```python
from build123d import *

# Parameters (mm, degrees)
F0_W     = 75.5904
F0_H     = 25.2222
F0_W_2   = 22.2504
F0_H_2   = 12.5222
F1_DEPTH = 0.9652
F2_W     = 31.75
F2_H     = 17.78
F3_DEPTH = 0.3048


with BuildPart() as f1:
    # F0 (on Top) → F1 (new body)
    with BuildSketch(Plane.XY):
        Rectangle(F0_W, F0_H)
        Rectangle(F0_W_2, F0_H_2, mode=Mode.SUBTRACT)
    extrude(amount=F1_DEPTH)

    # F2 (on face) → F3 (cut)
    with BuildSketch(Plane.XY.offset(0.9652)):
        Rectangle(F2_W, F2_H)
    extrude(amount=-F3_DEPTH, mode=Mode.SUBTRACT)


solid = f1.part
```
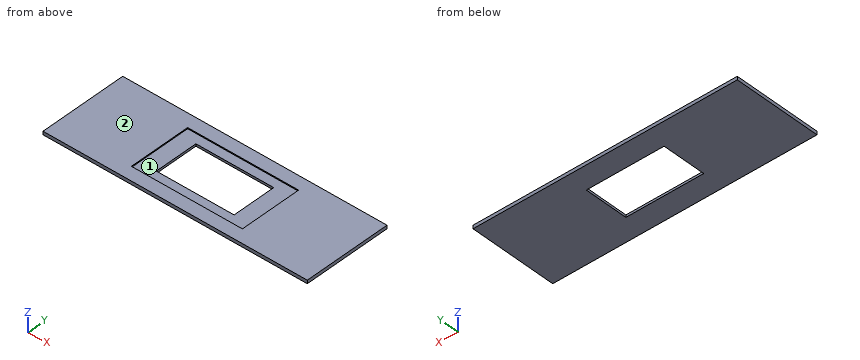
Verification items for the finished model (mm, model axes). Face numbers are marked on the shaded views. Round coordinates to 2 decimals unless told otherwise and drop trailing zeros. Order: outer loops, then holes, each group sorted by start corner. A loop starts at its lowest first (then second) coordinate and runs counter-clockwise, first axis right, second up. Notation, with made-up numbers: (-37.5, 76) -> (14.5, 76) arc R16 ccw to (14.5, 106) -> close; hole circle Ø5 at (12, -35). An arc over 180 degrees is marked (long way). Put each result on its own line as item: value. Start each with the question number.
(1) Depth check by flat-ended pin: pin 1 Ø1 at (x, y) = (-21, 0.5) entering from -Z. Enter the tip coordinate at first touch or a pass-through.
(2) Section check A-A (y = 2.75). Enter the section's corners in (x, z) (3 decimals), then the cut area to 3 significant figures.
(3) Draft check along Y on the marked faces 1 and 2. Enter one of: +Y half, -Y half, draft (parallel to the pull), parting line (faces both ways), or undercut.
(4) Section check D-D (x = 12). Enter the section's corners in (y, z), then the cut area to 3 significant figures.
(5) Material ranges on line 1 along X through (y, z) = (-5.75, 0.45); line 2 along X through (y, z) = (8.5, 0.85) (3 decimals); line 3 along Y through (x, z) = (1.5, 0.5), recorded low to high.
(6) Section check C-C (z = 0.5). Enter the section's corners in (x, y).
(7) Section check B-B (x = -1). Enter the section's corners in (y, z).
Completed:
1. pin 1: stops at z = 0
2. outline: (-37.795, 0) -> (-11.125, 0) -> (-11.125, 0.66) -> (-15.875, 0.66) -> (-15.875, 0.965) -> (-37.795, 0.965) -> close; (11.125, 0) -> (37.795, 0) -> (37.795, 0.965) -> (15.875, 0.965) -> (15.875, 0.66) -> (11.125, 0.66) -> close
2. area: 48.6 mm2
3. face 1: undercut
3. face 2: draft
4. outline: (-12.61, 0) -> (12.61, 0) -> (12.61, 0.97) -> (8.89, 0.97) -> (8.89, 0.66) -> (-8.89, 0.66) -> (-8.89, 0.97) -> (-12.61, 0.97) -> close
4. area: 18.9 mm2
5. line 1: x = -37.8 to -11.13, 11.13 to 37.8
5. line 2: x = -37.795 to -15.875, 15.875 to 37.795
5. line 3: y = -12.61 to -6.26, 6.26 to 12.61
6. outline: (-37.8, -12.61) -> (37.8, -12.61) -> (37.8, 12.61) -> (-37.8, 12.61) -> close; hole (-11.13, -6.26) -> (11.13, -6.26) -> (11.13, 6.26) -> (-11.13, 6.26) -> close
7. outline: (-12.61, 0) -> (-6.26, 0) -> (-6.26, 0.66) -> (-8.89, 0.66) -> (-8.89, 0.97) -> (-12.61, 0.97) -> close; (6.26, 0) -> (12.61, 0) -> (12.61, 0.97) -> (8.89, 0.97) -> (8.89, 0.66) -> (6.26, 0.66) -> close
